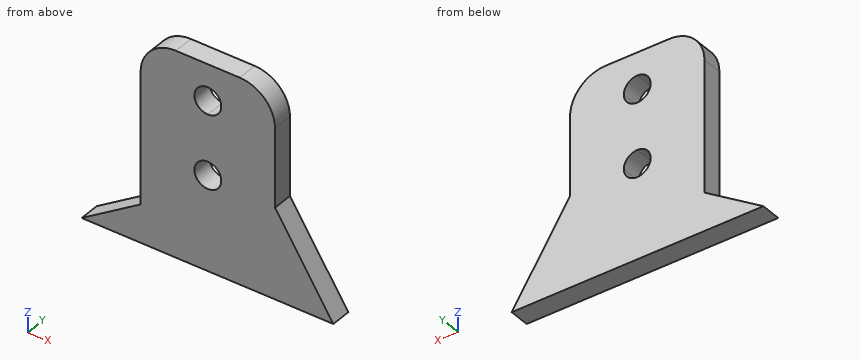
from build123d import *

# Parameters (mm, degrees)
F1_DEPTH = 3.5


with BuildPart() as f1:
    # F0 (on Front) → F1 (new body)
    with BuildSketch(Plane.XZ):
        with BuildLine():
            Line((0, 6.5), (0, 0))
            Line((0, 0), (23, 0))
            Line((23, 0), (23, 15.5))
            Line((23, 15.5), (23, 28.961353))
            ThreePointArc((23, 28.961353), (21.231321, 33.231321), (16.961353, 35))
            Line((16.961353, 35), (11.5, 35))
            Line((11.5, 35), (6.038647, 35))
            ThreePointArc((6.038647, 35), (1.768679, 33.231321), (0, 28.961353))
            Line((0, 28.961353), (0, 6.5))
        make_face()
        with BuildLine():
            ThreePointArc((13.8, 16.2), (9.873654, 14.573654), (11.5, 18.5))
            ThreePointArc((11.5, 18.5), (13.126346, 17.826346), (13.8, 16.2))
        make_face(mode=Mode.SUBTRACT)
        with BuildLine():
            ThreePointArc((11.5, 26.5), (9.2, 28.8), (11.5, 31.1))
            ThreePointArc((11.5, 31.1), (13.126346, 30.426346), (13.8, 28.8))
            ThreePointArc((13.8, 28.8), (13.126346, 27.173654), (11.5, 26.5))
        make_face(mode=Mode.SUBTRACT)
        Polygon((23, 15.5), (23, 0), (32.987984, 0), align=None)
        Polygon((-10.087121, 0), (0, 0), (0, 6.5), align=None)
    extrude(amount=F1_DEPTH)


solid = f1.part
For this review, take the finished solid that the model builds, in its own axes (mm). Give positions to 0.01 mm unless a question says otherwise; leave off trailing zeros. Order: outer loops, then holes, each group sorted by start corner. A loop starts at its lowest first (then second) coordinate and runs counter-clockwise, first axis right, second up. Notation, with made-up numbers: (79.25, 25.5) -> (96.25, 25.5) arc R24 ccw to (96.25, 54.5) -> close; hole circle Ø11 at (72.5, 86). An arc over 180 degrees is marked (long way). Write item = value, one per line.
1) We need section B-B, the plane z = 32. Give the boundary of the cut face in (x, y), and give its area (3 significant figures).
Findings:
outline = (0.82, -3.5) -> (22.18, -3.5) -> (22.18, 0) -> (0.82, 0) -> close
area = 74.8 mm^2
2) We need section C-C, the plane x = 29.5. Give the boundary of the cut face in (y, z).
Findings:
outline = (-3.5, 0) -> (0, 0) -> (0, 5.41) -> (-3.5, 5.41) -> close
3) To check wall thickness, follow L1, parallel to Z at x = 11.5, y = -2.6; L2, parallel to X at y = -1.85, z = 16.2; L3, parallel to X at y = -2.6, z = 30. State the ranges of each line that lie inside material, in increasing order. Write a range as from..to.
Findings:
L1 = 0..13.9, 18.5..26.5, 31.1..35
L2 = 0..9.2, 13.8..23
L3 = 0.09..9.54, 13.46..22.91
4) We need section A-A, the plane y = -0.45. Give the boundary of the cut face in (x, z).
Findings:
outline = (-10.09, 0) -> (32.99, 0) -> (23, 15.5) -> (23, 28.96) arc R6.04 ccw to (16.96, 35) -> (6.04, 35) arc R6.04 ccw to (0, 28.96) -> (0, 6.5) -> close; hole (11.5, 18.5) arc R2.3 ccw (long way) to (13.8, 16.2) arc R2.3 ccw to start; hole (11.5, 26.5) arc R2.3 ccw to (13.8, 28.8) arc R2.3 ccw to (11.5, 31.1) arc R2.3 ccw to start
5) Insertion check: pin 1 (1.8 mm diameter, centred on y = -1, z = 17.5, fed in from -X). The pin has a flat end and moves straight along its axis. Give the tip position at first contact, or say it passes through.
Findings:
pin_1 = 0
